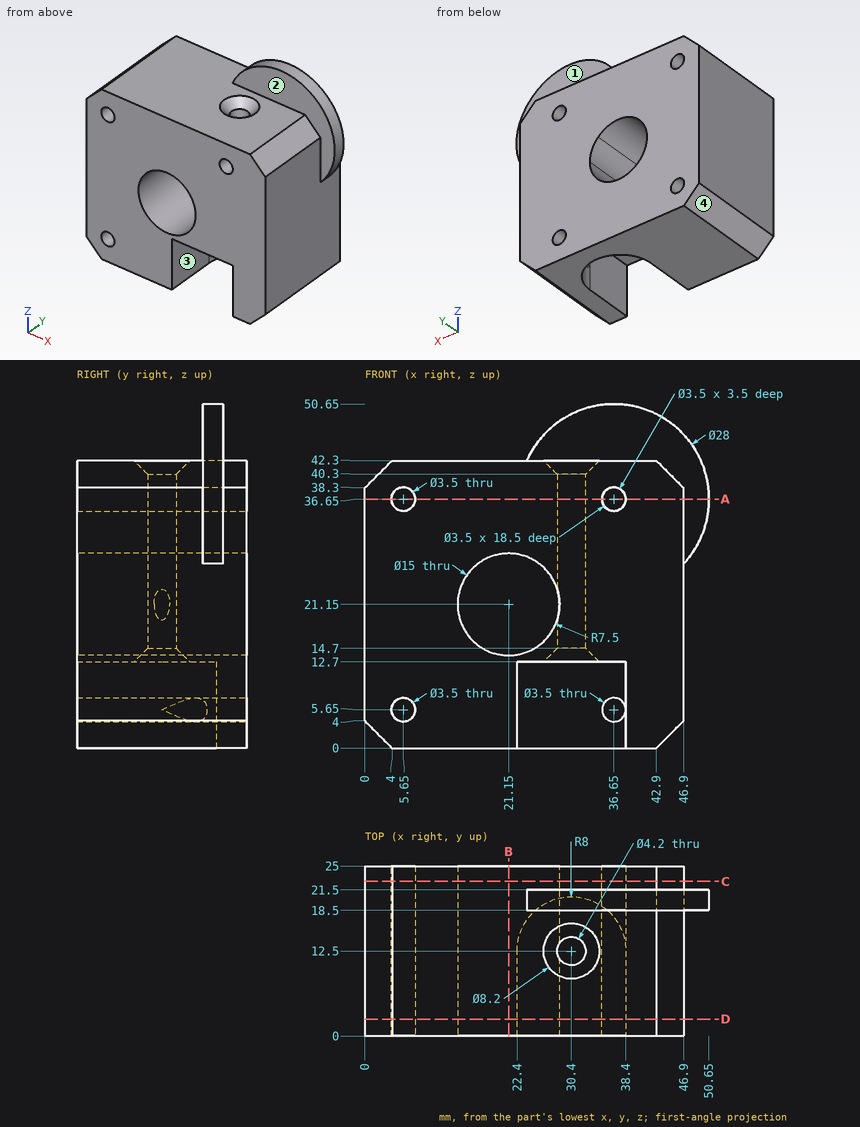
Can you work these out from the drawing? Everything is in mm from the part's minimum corner. A direction names the side the tool comes from. Round coordinates to 2 decimals unless told otherwise and drop trailing zeros. Loops run counter-clockwise (first coordinate to the right, second up) from the corner with the lowest first, then second, coordinate; pieces in that order, holes last. Notation, with made-up numbers: M 80.25,-18.75 L 104.25,-18.75 A18 cw 104.25,-2.75 Z; hole C -26.75,55 d7. An arc over 180 degrees is marked long. Write item = value, one per line.
1. Which directions (+Z, -Z, +X, -X, +Y, -Y) give clear straight access to the entire face, cutting with the end or side of a thin tool? Please do the marked faces 1, 2, 3 and 4.
Results below:
face_1 = +Z, +X, +Y
face_2 = +Z, +X, -Y
face_3 = -Z, -Y
face_4 = -Z, -X, +Y, -Y
2. Will these pins go through, and if not, where does the flat tip stop? P1, Ø1.5, axis at y = 19.5, z = 19, coming from the +X side; P2, Ø2, axis at x = 24, y = 12.5, coming from the +Z side; P3, Ø1.5, axis at x = 37, z = 45, coming from the +Y side.
Results below:
P1 = 46.9
P2 = 42.3
P3 = 21.5
3. I want a section at B-B, the plane x = 21.15. Write out the boundary of the cut face in (y, z), and give its area (4 significant figures).
Results below:
outline = M 0,0 L 25,0 L 25,13.65 L 0,13.65 Z; M 0,28.65 L 25,28.65 L 25,42.3 L 0,42.3 Z
area = 682.5 mm²
4. I want a section at D-D, the plane y = 2.5. Write out the boundary of the cut face in (x, z), and give its area (3 significant figures).
Results below:
outline = M 0,4 L 4,0 L 22.4,0 L 22.4,12.7 L 38.4,12.7 L 38.4,0 L 42.9,0 L 46.9,4 L 46.9,38.3 L 42.9,42.3 L 4,42.3 L 0,38.3 Z; hole C 5.65,5.65 d3.5; hole C 5.65,36.65 d3.5; hole C 21.15,21.15 d15; hole C 36.65,36.65 d3.5
area = 1,540 mm²
5. I want a section at C-C, the plane y = 22.75. Write out the boundary of the cut face in (x, z), and give its area (3 significant figures).
Results below:
outline = M 0,4 L 4,0 L 42.9,0 L 46.9,4 L 46.9,38.3 L 42.9,42.3 L 4,42.3 L 0,38.3 Z; hole C 5.65,5.65 d3.5; hole C 5.65,36.65 d3.5; hole C 21.15,21.15 d15; hole C 36.65,5.65 d3.5; hole C 36.65,36.65 d3.5
area = 1,740 mm²
6. I want a section at A-A, the plane z = 36.65. Write out the boundary of the cut face in (x, y), and give its area (3 significant figures).
Results below:
outline = M 0,0 L 3.9,0 L 3.9,25 L 0,25 Z; M 7.4,0 L 34.9,0 L 34.9,18.5 L 38.4,18.5 L 38.4,0 L 46.9,0 L 46.9,18.5 L 50.65,18.5 L 50.65,21.5 L 46.9,21.5 L 46.9,25 L 38.4,25 L 38.4,21.5 L 34.9,21.5 L 34.9,25 L 7.4,25 Z; hole C 30.4,12.5 d4.2
area = 1,010 mm²
7. I need wall thicknesses on probe 1 along Z at (x, y) = (5.65, 11.5); probe 2 along Z at (x, y) = (36.5, 11.25); probe 3 along Y at (x, z) = (30.4, 23.75). Which ranges of each line are inside material? Lowest first, please.
Results below:
probe_1 = 0 to 3.9, 7.4 to 34.9, 38.4 to 42.3
probe_2 = 12.7 to 34.91, 38.39 to 42.3
probe_3 = 0 to 10.4, 14.6 to 25
